```python
from build123d import *

# Parameters (mm, degrees)
F0_W      = 170
F0_H      = 15
F1_DEPTH  = 150
F2_W      = 170
F2_H      = 20
F3_DEPTH  = 5
F4_R      = 20
F5_DEPTH  = 25
F7_D      = 7
F8_DEPTH  = 5
F9_DEPTH  = 5
F11_D     = 7
F13_D     = 7
F14_DEPTH = 20
F16_D     = 7


# Not quite as in the source:
# - a feature names something its author has since deleted; it is built from what else it names


with BuildPart() as f1:
    # F0 (on Front) → F1 (new body)
    with BuildSketch(Plane.XZ):
        with Locations((85, 7.5)):
            Rectangle(F0_W, F0_H)
    extrude(amount=F1_DEPTH)

    # F2 (on face) → F3 (cut)
    with BuildSketch(Plane(origin=(0, 0, 0), x_dir=(1, 0, 0), z_dir=(0, 0, -1))):
        with Locations((85, 95)):
            Rectangle(F2_W, F2_H)
    extrude(amount=-F3_DEPTH, mode=Mode.SUBTRACT)

    # F4 (on face) → F5 (cut)
    with BuildSketch(Plane.XY.offset(15)):
        with Locations((85, -55)):
            Circle(F4_R)
    extrude(amount=-F5_DEPTH, mode=Mode.SUBTRACT)

    # F7 (through all)
    with Locations(Plane.XY.offset(15)):
        with Locations((61.5, -31.5), (61.5, -78.5), (108.5, -78.5), (108.5, -31.5)):
            Hole(F7_D / 2)

    # F8 (add): a face of the model
    f8_faces = [f1.faces().sort_by_distance(p)[0] for p in [
        (0, -74.0697674419, 7.7325581395),
    ]]
    extrude(f8_faces, amount=F8_DEPTH)

    # F9 (add): a face of the model
    f9_faces = [f1.faces().sort_by_distance(p)[0] for p in [
        (170, -74.0697674419, 7.7325581395),
    ]]
    extrude(f9_faces, amount=F9_DEPTH)

    # F11 (through all)
    with Locations(Plane.XY.offset(15)):
        with Locations((50, -95), (15, -95), (85, -95), (120, -95), (155, -95)):
            Hole(F11_D / 2)

    # F13 (through all)
    with Locations(Plane.XY.offset(15)):
        with Locations((10, -120), (160, -120)):
            Hole(F13_D / 2)

    # F14 (add): a face of the model
    f14_faces = [f1.faces().sort_by_distance(p)[0] for p in [
        (85, -150, 7.5),
    ]]
    extrude(f14_faces, amount=F14_DEPTH)

    # F16 (through all)
    with Locations(Plane.XY.offset(15)):
        with Locations((10, -150), (160, -150)):
            Hole(F16_D / 2)


solid = f1.part
```
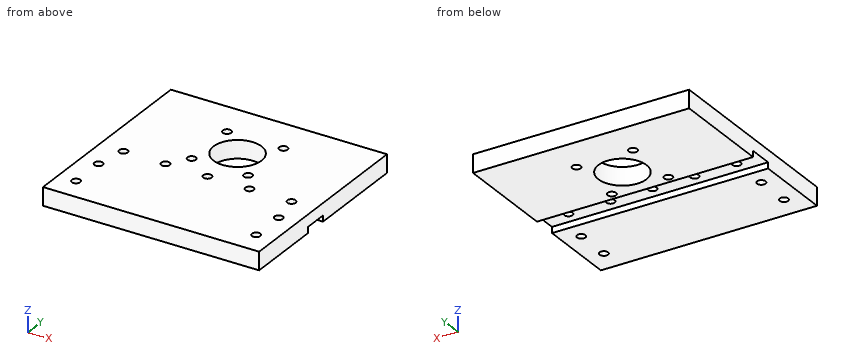
Model file for the job. Use its own axes, mm. Coordinates: 2 decimals unless noted, no trailing zeros. Loops run counter-clockwise (first coordinate to the right, second up) from the corner with the lowest first, then second, coordinate; pieces in that order, holes last. Notation, with made-up numbers: (-9.75, 65.5) -> (33.25, 65.5) arc R20 cw to (33.25, 69.5) -> close; hole circle Ø3 at (74.5, -9.75). An arc over 180 degrees is marked (long way). Answer as a JSON object with one key per item and string values.
Q1. Cut at C-C (y = -95). List the corners of the cut face in (x, z), and give its area (3 significant figures).
Report:
{"outline": "(-5, 5) -> (11.5, 5) -> (11.5, 15) -> (-5, 15) -> close; (18.5, 5) -> (46.5, 5) -> (46.5, 15) -> (18.5, 15) -> close; (53.5, 5) -> (81.5, 5) -> (81.5, 15) -> (53.5, 15) -> close; (88.5, 5) -> (116.5, 5) -> (116.5, 15) -> (88.5, 15) -> close; (123.5, 5) -> (151.5, 5) -> (151.5, 15) -> (123.5, 15) -> close; (158.5, 5) -> (175, 5) -> (175, 15) -> (158.5, 15) -> close", "area": "1,450 mm2"}
Q2. Flat gauge pins, fed straight in: P1, Ø5.5, axis at x = 61.5, y = -31.5, coming from the +Z side; P2, Ø10, axis at x = 124.5, y = -97.5, coming from the -Z side. Where does each tip first touch, or does it go through?
Report:
{"P1": "passes through", "P2": "stops at z = 5"}
Q3. Cut at A-A (x = 85). List the corners of the cut face in (y, z), and give its area (3 significant figures).
Report:
{"outline": "(-170, 0) -> (-105, 0) -> (-105, 5) -> (-98.5, 5) -> (-98.5, 15) -> (-170, 15) -> close; (-91.5, 5) -> (-85, 5) -> (-85, 0) -> (-75, 0) -> (-75, 15) -> (-91.5, 15) -> close; (-35, 0) -> (0, 0) -> (0, 15) -> (-35, 15) -> close", "area": "1,780 mm2"}
Q4. Cut at B-B (y = -150). List the corners of the cut face in (x, z).
Report:
{"outline": "(-5, 0) -> (6.5, 0) -> (6.5, 15) -> (-5, 15) -> close; (13.5, 0) -> (156.5, 0) -> (156.5, 15) -> (13.5, 15) -> close; (163.5, 0) -> (175, 0) -> (175, 15) -> (163.5, 15) -> close"}
Q5. Cut at D-D (z = 12). State how many separate pieces and enclosed holes the cut face has, and give its area (3 significant figures).
Report:
{"separate pieces": "1", "enclosed holes": "14", "area": "28,800 mm2"}
Q6. Probe probe 1 along X at (y, z) = (-78, 7.25); probe 2 along Y at (x, z) = (85, 7.5); probe 3 along Y at (x, z) = (85, 4.5). List the from-to ranges inside material, lowest first.
Report:
{"probe 1": "x = -5 to 58.04, 64.96 to 105.04, 111.96 to 175", "probe 2": "y = -170 to -98.5, -91.5 to -75, -35 to 0", "probe 3": "y = -170 to -105, -85 to -75, -35 to 0"}
